Source: CAD feature listing. Evaluate the final solid. Frame: model axes, mm. A direction names the side the tool comes from. Round coordinates to 2 decimals unless told otherwise and drop trailing zeros. Order: outer loops, then holes, each group sorted by start corner. A loop starts at its lowest first (then second) coordinate and runs counter-clockwise, first axis right, second up. Notation, with made-up numbers: (28, 80) - (52, 80) arc R33 cw to (52, 117) - close; hole circle Ø5 at (29.5, -15.75). An arc over 180 degrees is marked (long way). Use one line per item in the form item = value. Start each with the question number.
Q1. Ray query, line 1 (Y direction, x = -16.5, z = 12); line 2 (Z direction, x = 6.5, y = -30.5); line 3 (Z direction, x = 0, y = 10). Return the intervals inside material, ascending. Write a range as [from, to].
Q2. Draft query along X for faces 6 (the flat face through (0, 2, -6.5)), 7 (the flat face through (12.5, -19, 27)), 8 (the flat face through (0, -26, -26)). Return one class per face: released by +X, released by -X, zero draft, split by the parting line, or undercut.
Q3. Cut plane B-B, the plane z = -23.5. Return the cut outline in (x, y), and give its area (3 significant figures).
Q4. Pin query (flat end, axial travel): pin 1 Ø10 at (x, z) = (3.5, 3) entering from -Y; pin 2 Ø1.1 at (y, z) = (-38, -26.5) entering from -X; pin 3 Ø12.5 at (x, y) = (3, -35.5) entering from -Z. Return the tip coordinate at first contact, or that it passes through.
Q5. Cut plane D-D, the plane x = 0. Give the number of separate pieces and of enclosed holes in the cut face, and give its area (3 significant figures).
Q6. Set-up query: faces 1 (the cylindrical face through (0, -16.1, -22.8)), 2 (the flat face through (4.1, 1, -10)), 3 (the flat face through (12.5, -19, -27)), 4 (the cylindrical face through (-2.343, 9.86, -17.847)), 5 (the flat face through (8, 7, -18)). Return all of +Z, -Z, +X, -X, +Y, -Y with unobstructed straight access to the full face (end or side cutting, diameter ignored); none if empty.
Q7. Cut plane C-C, the plane y = -6. Return the cut outline in (x, z), and give its area (3 significant figures).
Q8. Cut plane A-A, the plane y = -32. Return the cut outline in (x, z), and give its area (3 significant figures).
from build123d import *

# Parameters (mm, degrees)
SKETCH_1_R           = 19.5
SKETCH_1_R_2         = 18
EXTRUDE_1_DEPTH      = 20
SKETCH_3_R           = 27.5
EXTRUDE_2_DEPTH      = 3
SKETCH_25_R          = 21.75
SKETCH_25_R_2        = 19.5
EXTRUDE_12_DEPTH     = 2
EXTRUDE_START        = -1
SKETCH_26_R          = 21.75
SKETCH_26_R_2        = 19.5
EXTRUDE_13_DEPTH     = 2
EXTRUDE_14_DEPTH     = 3
SKETCH_28_W          = 21.458236
SKETCH_28_H          = 3
SKETCH_28_W_2        = 3.541764
EXTRUDE_17_DEPTH     = 1.5
EXTRUDE_25_DEPTH     = 53.5
CUT_EXTRUDE_15_DEPTH = 52
EXTRUDE_24_DEPTH     = 3
EXTRUDE_23_DEPTH     = 8
SKETCH_38_3_R        = 4.8
CUT_EXTRUDE_10_DEPTH = 9.5
SKETCH_34_W          = 10.2
SKETCH_34_H          = 6.5
SKETCH_34_W_2        = 8.2
SKETCH_34_H_2        = 4.5
EXTRUDE_22_DEPTH     = 5
SKETCH_37_W          = 8.2
SKETCH_37_H          = 4.5
CUT_EXTRUDE_9_DEPTH  = 5


with BuildPart() as part:
    # Sketch 1 → Extrude 1 (new body)
    with BuildSketch(Plane(origin=(0, 0, 0), x_dir=(1, 0, 0), z_dir=(0, 1, 0))):
        Circle(SKETCH_1_R)
        Circle(SKETCH_1_R_2, mode=Mode.SUBTRACT)
    extrude(amount=EXTRUDE_1_DEPTH)

    # Sketch 3 → Extrude 2 (add)
    with BuildSketch(Plane.XZ):
        Circle(SKETCH_3_R)
    extrude(amount=EXTRUDE_2_DEPTH)

    # Sketch 25 → Extrude 12 (add)
    with BuildSketch(Plane(origin=(0, 7, 0), x_dir=(-1, 0, 0), z_dir=(0, -1, 0))):
        Circle(SKETCH_25_R)
        Circle(SKETCH_25_R_2, mode=Mode.SUBTRACT)
    extrude(amount=EXTRUDE_12_DEPTH)

    # Sketch 26 → Extrude 13 (add)
    with BuildSketch(Plane(origin=(0, 10.5, 0), x_dir=(-1, 0, 0), z_dir=(0, -1, 0)).offset(EXTRUDE_START)):
        Circle(SKETCH_26_R)
        Circle(SKETCH_26_R_2, mode=Mode.SUBTRACT)
    extrude(amount=-EXTRUDE_13_DEPTH)

    # Sketch 27 → Extrude 14 (add)
    with BuildSketch(Plane.XZ.offset(3)):
        with BuildLine():
            Line((-12.5, 27.5), (-12.5, 24.494897))
            ThreePointArc((-12.5, 24.494897), (-6.428076, 26.738172), (0, 27.5))
            Line((0, 27.5), (-12.5, 27.5))
        make_face()
        with BuildLine():
            ThreePointArc((-8.958236, -26), (-10.755478, -25.309478), (-12.5, -24.494897))
            Line((-12.5, -24.494897), (-12.5, -26))
            Line((-12.5, -26), (-8.958236, -26))
        make_face()
        with BuildLine():
            ThreePointArc((0, 27.5), (6.428076, 26.738172), (12.5, 24.494897))
            Line((12.5, 24.494897), (12.5, 27.5))
            Line((12.5, 27.5), (0, 27.5))
        make_face()
        with BuildLine():
            Line((12.5, -26), (12.5, -24.494897))
            ThreePointArc((12.5, -24.494897), (10.755478, -25.309478), (8.958236, -26))
            Line((8.958236, -26), (12.5, -26))
        make_face()
    extrude(amount=-EXTRUDE_14_DEPTH)

    # Sketch 28 → Extrude 17 (add)
    with BuildSketch(Plane(origin=(0, 0, -26), x_dir=(-1, 0, 0), z_dir=(0, 0, -1))):
        with BuildLine():
            Line((12.5, -38), (12.5, -3))
            Line((12.5, -3), (8.958236, -3))
            Line((8.958236, -3), (-12.5, -3))
            Line((-12.5, -3), (-12.5, -38))
            Line((-12.5, -38), (-8.6, -38))
            Line((-8.6, -38), (-8.6, -37.5))
            ThreePointArc((-8.6, -37.5), (-7.1, -36), (-5.6, -37.5))
            Line((-5.6, -37.5), (-5.6, -38))
            Line((-5.6, -38), (-4, -38))
            ThreePointArc((-4, -38), (0, -34), (4, -38))
            Line((4, -38), (5.6, -38))
            Line((5.6, -38), (5.6, -37.5))
            ThreePointArc((5.6, -37.5), (7.1, -36), (8.6, -37.5))
            Line((8.6, -37.5), (8.6, -38))
            Line((8.6, -38), (12.5, -38))
        make_face()
        with Locations((-1.770882, -1.5)):
            Rectangle(SKETCH_28_W, SKETCH_28_H)
        with Locations((10.729118, -1.5)):
            Rectangle(SKETCH_28_W_2, SKETCH_28_H)
        with BuildLine():
            ThreePointArc((-12.5, -38), (0, -50.5), (12.5, -38))
            Line((12.5, -38), (8.6, -38))
            Line((8.6, -38), (8.6, -38.5))
            ThreePointArc((8.6, -38.5), (7.1, -40), (5.6, -38.5))
            Line((5.6, -38.5), (5.6, -38))
            Line((5.6, -38), (4, -38))
            ThreePointArc((4, -38), (0, -42), (-4, -38))
            Line((-4, -38), (-5.6, -38))
            Line((-5.6, -38), (-5.6, -38.5))
            ThreePointArc((-5.6, -38.5), (-7.1, -40), (-8.6, -38.5))
            Line((-8.6, -38.5), (-8.6, -38))
            Line((-8.6, -38), (-12.5, -38))
        make_face()
    extrude(amount=EXTRUDE_17_DEPTH)

    # Sketch 28_25 → Extrude 25 (add)
    with BuildSketch(Plane(origin=(0, 0, -26), x_dir=(-1, 0, 0), z_dir=(0, 0, -1))):
        with BuildLine():
            Line((12.5, -38), (12.5, -3))
            Line((12.5, -3), (8.958236, -3))
            Line((8.958236, -3), (-12.5, -3))
            Line((-12.5, -3), (-12.5, -38))
            Line((-12.5, -38), (-8.6, -38))
            Line((-8.6, -38), (-8.6, -37.5))
            ThreePointArc((-8.6, -37.5), (-7.1, -36), (-5.6, -37.5))
            Line((-5.6, -37.5), (-5.6, -38))
            Line((-5.6, -38), (-4, -38))
            ThreePointArc((-4, -38), (0, -34), (4, -38))
            Line((4, -38), (5.6, -38))
            Line((5.6, -38), (5.6, -37.5))
            ThreePointArc((5.6, -37.5), (7.1, -36), (8.6, -37.5))
            Line((8.6, -37.5), (8.6, -38))
            Line((8.6, -38), (12.5, -38))
        make_face()
        with BuildLine():
            ThreePointArc((-12.5, -38), (0, -50.5), (12.5, -38))
            Line((12.5, -38), (8.6, -38))
            Line((8.6, -38), (8.6, -38.5))
            ThreePointArc((8.6, -38.5), (7.1, -40), (5.6, -38.5))
            Line((5.6, -38.5), (5.6, -38))
            Line((5.6, -38), (4, -38))
            ThreePointArc((4, -38), (0, -42), (-4, -38))
            Line((-4, -38), (-5.6, -38))
            Line((-5.6, -38), (-5.6, -38.5))
            ThreePointArc((-5.6, -38.5), (-7.1, -40), (-8.6, -38.5))
            Line((-8.6, -38.5), (-8.6, -38))
            Line((-8.6, -38), (-12.5, -38))
        make_face()
    extrude(amount=-EXTRUDE_25_DEPTH)

    # Sketch 28_27 → Cut-Extrude 15 (cut)
    with BuildSketch(Plane(origin=(0, 0, -26), x_dir=(-1, 0, 0), z_dir=(0, 0, -1))):
        with BuildLine():
            ThreePointArc((-12.5, -38), (0, -50.5), (12.5, -38))
            Line((12.5, -38), (8.6, -38))
            Line((8.6, -38), (8.6, -38.5))
            ThreePointArc((8.6, -38.5), (7.1, -40), (5.6, -38.5))
            Line((5.6, -38.5), (5.6, -38))
            Line((5.6, -38), (4, -38))
            ThreePointArc((4, -38), (0, -42), (-4, -38))
            Line((-4, -38), (-5.6, -38))
            Line((-5.6, -38), (-5.6, -38.5))
            ThreePointArc((-5.6, -38.5), (-7.1, -40), (-8.6, -38.5))
            Line((-8.6, -38.5), (-8.6, -38))
            Line((-8.6, -38), (-12.5, -38))
        make_face()
        with BuildLine():
            Line((12.5, -38), (12.5, -3))
            Line((12.5, -3), (8.958236, -3))
            Line((8.958236, -3), (-12.5, -3))
            Line((-12.5, -3), (-12.5, -38))
            Line((-12.5, -38), (-8.6, -38))
            Line((-8.6, -38), (-8.6, -37.5))
            ThreePointArc((-8.6, -37.5), (-7.1, -36), (-5.6, -37.5))
            Line((-5.6, -37.5), (-5.6, -38))
            Line((-5.6, -38), (-4, -38))
            ThreePointArc((-4, -38), (0, -34), (4, -38))
            Line((4, -38), (5.6, -38))
            Line((5.6, -38), (5.6, -37.5))
            ThreePointArc((5.6, -37.5), (7.1, -36), (8.6, -37.5))
            Line((8.6, -37.5), (8.6, -38))
            Line((8.6, -38), (12.5, -38))
        make_face()
    extrude(amount=-CUT_EXTRUDE_15_DEPTH, mode=Mode.SUBTRACT)

    # Sketch 38_4 → Extrude 24 (add)
    with BuildSketch(Plane(origin=(0, 0, -27.5), x_dir=(-1, 0, 0), z_dir=(0, 0, -1))):
        with BuildLine():
            Line((-1.3125, -15.961765), (-1, -14.494678))
            ThreePointArc((-1, -14.494678), (-3.019934, -6.069048), (4.8, -9.8))
            ThreePointArc((4.8, -9.8), (3.730952, -12.819934), (1, -14.494678))
            Line((1, -14.494678), (1.3125, -15.961765))
            ThreePointArc((1.3125, -15.961765), (4.896874, -13.763663), (6.3, -9.8))
            ThreePointArc((6.3, -9.8), (-3.963663, -4.903126), (-1.3125, -15.961765))
        make_face()
    extrude(amount=EXTRUDE_24_DEPTH)

    # Sketch 38 → Extrude 23 (add)
    with BuildSketch(Plane(origin=(0, 0, -27.5), x_dir=(-1, 0, 0), z_dir=(0, 0, -1))):
        with BuildLine():
            ThreePointArc((1, -14.494678), (0, -14.6), (-1, -14.494678))
            Line((-1, -14.494678), (-1.3125, -15.961765))
            ThreePointArc((-1.3125, -15.961765), (0, -16.1), (1.3125, -15.961765))
            Line((1.3125, -15.961765), (1, -14.494678))
        make_face()
        with BuildLine():
            Line((-1.3125, -15.961765), (-1, -14.494678))
            ThreePointArc((-1, -14.494678), (-3.019934, -6.069048), (4.8, -9.8))
            ThreePointArc((4.8, -9.8), (3.730952, -12.819934), (1, -14.494678))
            Line((1, -14.494678), (1.3125, -15.961765))
            ThreePointArc((1.3125, -15.961765), (4.896874, -13.763663), (6.3, -9.8))
            ThreePointArc((6.3, -9.8), (-3.963663, -4.903126), (-1.3125, -15.961765))
        make_face()
    extrude(amount=-EXTRUDE_23_DEPTH)

    # Sketch 38_3 → Cut-Extrude 10 (cut)
    with BuildSketch(Plane(origin=(0, 0, -27.5), x_dir=(-1, 0, 0), z_dir=(0, 0, -1))):
        with Locations((0, -9.8)):
            Circle(SKETCH_38_3_R)
    extrude(amount=-CUT_EXTRUDE_10_DEPTH, mode=Mode.SUBTRACT)

    # Sketch 34 → Extrude 22 (add)
    with BuildSketch(Plane(origin=(0, 0, 0), x_dir=(1, 0, 0), z_dir=(0, 1, 0))):
        with Locations((0, 9.75)):
            Rectangle(SKETCH_34_W, SKETCH_34_H)
        with Locations((0, 9.75)):
            Rectangle(SKETCH_34_W_2, SKETCH_34_H_2, mode=Mode.SUBTRACT)
    extrude(amount=EXTRUDE_22_DEPTH)

    # Sketch 37 → Cut-Extrude 9 (cut)
    with BuildSketch(Plane(origin=(0, 0, 0), x_dir=(1, 0, 0), z_dir=(0, 1, 0))):
        with Locations((0, 9.75)):
            Rectangle(SKETCH_37_W, SKETCH_37_H)
    extrude(amount=-CUT_EXTRUDE_9_DEPTH, mode=Mode.SUBTRACT)


solid = part.part
Completed:
q1.line_1 = [-3, 0], [5, 7], [11.5, 13.5]
q1.line_2 = [-27.5, -26], [26, 27.5]
q1.line_3 = [-19.5, -18], [18, 19.5]
q2.face_6 = undercut
q2.face_7 = released by +X
q2.face_8 = zero draft
q3.outline = (-14.28, -3) - (14.28, -3) - (14.28, 0) - (-14.28, 0) - close; (-1.31, -15.96) arc R6.3 ccw to (1.31, -15.96) arc R6.3 ccw (long way) to start; hole (-4.8, -9.8) arc R4.8 ccw to (-1, -14.49) arc R4.8 ccw to (1, -14.49) arc R4.8 ccw (long way) to start
q3.area = 138 mm2
q4.pin_1 = -3
q4.pin_2 = -12.5
q4.pin_3 = -27.5
q5.separate_pieces = 5
q5.enclosed_holes = 0
q5.area = 368 mm2
q6.face_1 = -Y
q6.face_2 = +Y, -Y
q6.face_3 = -Z, +X, +Y, -Y
q6.face_4 = +Y
q6.face_5 = none
q7.outline = (-12.5, -27.5) - (-5.02, -27.5) - (-5.02, -30.5) - (-2.93, -30.5) - (-2.93, -19.5) - (-5.02, -19.5) - (-5.02, -26) - (-12.5, -26) - close; (-12.5, 26) - (12.5, 26) - (12.5, 27.5) - (-12.5, 27.5) - close; (2.93, -30.5) - (5.02, -30.5) - (5.02, -27.5) - (12.5, -27.5) - (12.5, -26) - (5.02, -26) - (5.02, -19.5) - (2.93, -19.5) - (2.93, -26) - close
q7.area = 106 mm2
q8.outline = (-12.5, -27.5) - (12.5, -27.5) - (12.5, -26) - (-12.5, -26) - close; (-12.5, 26) - (12.5, 26) - (12.5, 27.5) - (-12.5, 27.5) - close
q8.area = 75.0 mm2
